```python
from build123d import *

# Parameters (mm, degrees)
SKETCH1_R           = 1.2192
BOSS_EXTRUDE1_DEPTH = 5.842


with BuildPart() as part:
    # Sketch1 → Boss-Extrude1 (new body)
    with BuildSketch(Plane.XY):
        with BuildLine():
            Line((12.7, 32.629483496), (12.7, 0))
            ThreePointArc((12.7, 0), (0, -12.7), (-12.7, 0))
            Line((-12.7, 0), (-12.7, 32.629483496))
            ThreePointArc((-12.7, 32.629483496), (-19.764825615, -28.901987157), (35.0139, 0))
            ThreePointArc((35.0139, 0), (28.901987157, 19.764825615), (12.7, 32.629483496))
        make_face()
        with Locations((0, -25.4)):
            Circle(SKETCH1_R, mode=Mode.SUBTRACT)
        with Locations((-25.4, 0)):
            Circle(SKETCH1_R, mode=Mode.SUBTRACT)
        with Locations((25.4, 0)):
            Circle(SKETCH1_R, mode=Mode.SUBTRACT)
    extrude(amount=BOSS_EXTRUDE1_DEPTH)


solid = part.part
```
Can you work these out from the model? Positions are in its coordinate system, mm. A direction names the side the tool comes from. Give positions to 0.01 mm unless a question says otherwise; leave off trailing zeros. Order: outer loops, then holes, each group sorted by start corner. A loop starts at its lowest first (then second) coordinate and runs counter-clockwise, first axis right, second up. Notation, with made-up numbers: (59.5, 38) - (92.5, 38) arc R14 cw to (92.5, 60) - close; hole circle Ø4 at (74.5, 14.25). An arc over 180 degrees is marked (long way). Use a Markdown table: item, result. Add a question column.
Q1. On a 3-axis mill with a long thin cutter (end or side, diameter ignored), from which of +Z, -Z, +X, -X, +Y, -Y can I reach the whole of each face in a straight line? I mean faces 3 (the flat face through (-12.7, 16, 3)), 4 (the cylindrical face through (26.56, 0.37, 2.88)). Say none if no direction works.
Q2. I'm going to push flat-ended pins straight in: pin 1 (3 mm diameter, centred on y = -11.5, z = 2.5, fed in from +X); pin 2 (10 mm diameter, centred on x = -27, y = 25, fed in from -Z); pin 3 (1.8 mm diameter, centred on y = 24, z = 3.5, fed in from -X); pin 4 (2 mm diameter, centred on y = -2.5, z = 3, fed in from +X). Where does each tip first touch, or does it pass through?
Q3. Please list where these lines run through material, in increasing order: line 1 along Y through (x, z) = (0, 1.85); line 2 along X through (y, z) = (-26, 0.45); line 3 along X through (y, z) = (22, 0.6).
Q4. If we section it at D-D on x = -14: Write out the boundary of the cut face in (y, z).
Q5. If we section it at C-C on y = 11: Write out the boundary of the cut face in (x, z), plus the area to 3 significant figures.
Q6. If we section it at B-B on z = 4.65: Write out the boundary of the cut face in (x, y).
Q7. If we mould it in two halves opening along X, with no side actions, what happens to faces 1 (the flat face through (0, -16, 0)), 2 (the flat face through (12.7, 17, 3))? For each: released by +X, released by -X, zero draft, split by the parting line, or undercut.
Q8. If we section it at A-A on x = 0: Write out the boundary of the cut face in (y, z).
Answers follow:
| question | item | result |
|---|---|---|
| 1 | face 3 | +Z, -Z, +Y |
| 1 | face 4 | +Z, -Z |
| 2 | pin 1 | stops at x = 33.56 |
| 2 | pin 2 | stops at z = 0 |
| 2 | pin 3 | stops at x = -26.31 |
| 2 | pin 4 | stops at x = 34.98 |
| 3 | line 1 | y = -35.01 to -26.62, -24.18 to -12.7 |
| 3 | line 2 | x = -23.45 to -1.06, 1.06 to 23.45 |
| 3 | line 3 | x = -27.24 to -12.7, 12.7 to 27.24 |
| 4 | outline | (-32.09, 0) - (32.09, 0) - (32.09, 5.84) - (-32.09, 5.84) - close |
| 5 | outline | (-33.24, 0) - (-12.7, 0) - (-12.7, 5.84) - (-33.24, 5.84) - close; (12.7, 0) - (33.24, 0) - (33.24, 5.84) - (12.7, 5.84) - close |
| 5 | area | 240 mm^2 |
| 6 | outline | (-12.7, 0) - (-12.7, 32.63) arc R35.01 ccw (long way) to (12.7, 32.63) - (12.7, 0) arc R12.7 cw to start; hole circle Ø2.44 at (-25.4, 0); hole circle Ø2.44 at (0, -25.4); hole circle Ø2.44 at (25.4, 0) |
| 7 | face 1 | zero draft |
| 7 | face 2 | undercut |
| 8 | outline | (-35.01, 0) - (-26.62, 0) - (-26.62, 5.84) - (-35.01, 5.84) - close; (-24.18, 0) - (-12.7, 0) - (-12.7, 5.84) - (-24.18, 5.84) - close |
